Source: CAD feature listing. Evaluate the final solid. Frame: model axes, mm. Face numbers are marked on the shaded views. A direction names the side the tool comes from. Round coordinates to 2 decimals unless told otherwise and drop trailing zeros. Loops run counter-clockwise (first coordinate to the right, second up) from the corner with the lowest first, then second, coordinate; pieces in that order, holes last.
(1) Material intervals for probe 1 along X at (y, z) = (300, 0.75); probe 2 along Y at (x, z) = (4, 0.45); probe 3 along X at (y, z) = (301, 2.05), sorted ascending.
(2) Section A-A, the plane x = 4. Return the cut outline in (y, z), plus the area to 3 significant figures.
(3) Section B-B, the plane z = 2.75. Return the cut outline in (x, y) (3 decimals).
(4) First-contact query: pin 1 Ø4.5 at (x, y) = (2.5, 300) entering from +Z; pin 2 Ø1.7 at (x, y) = (-3, 300) entering from +Z. Flat tips, straight axial feed; report the tip coordinate or a pass-through.
(5) Section D-D, the plane x = 6.25. Return the cut outline in (y, z).
(6) Set-up query: the marked faces 1 and 2. Return all of +Z, -Z, +X, -X, +Y, -Y with unobstructed straight access to the full face (end or side cutting, diameter ignored); none if empty.
(7) Section C-C, the plane y = 298.75. Return the cut outline in (x, z), plus the area to 3 significant figures.
(8) Mould query, pull axis X, two halves, no side actions, for the marked faces 3, 4 and 5. Classes: pulls with the +X half, pulls with the -X half, needs draft (parallel to the pull), parting line crosses it, or undercut.
```python
from build123d import *

# Parameters (mm, degrees)
SKETCH_1_W                  = 18
SKETCH_1_H                  = 8
EXTRUDE_1_DEPTH             = 3
CUT_EXTRUDE_1_DEPTH         = 2
CUT_EXTRUDE_2_DEPTH         = 2
HOLE_WIZARD_3_6_3_6_1_D     = 3.6
HOLE_WIZARD_3_6_3_6_1_DEPTH = 3


with BuildPart() as part:
    # 草图1 → 凸台-拉伸1 (new body)
    with BuildSketch(Plane(origin=(0, 0, 0), x_dir=(-1, 0, 0), z_dir=(0, 0, -1))):
        with Locations((0, 300)):
            Rectangle(SKETCH_1_W, SKETCH_1_H)
    extrude(amount=-EXTRUDE_1_DEPTH)

    # 草图2 → 切除-拉伸1 (cut)
    with BuildSketch(Plane.XY.offset(3)):
        Polygon((-0.65, 300), (-2.325, 302.901185103), (-5.675, 302.901185103), (-7.35, 300), (-5.675, 297.098814897), (-2.325, 297.098814897), align=None)
    extrude(amount=-CUT_EXTRUDE_1_DEPTH, mode=Mode.SUBTRACT)

    # 草图3 → 切除-拉伸2 (cut)
    with BuildSketch(Plane.XY.offset(3)):
        Polygon((5.675, 297.098814897), (7.35, 300), (5.675, 302.901185103), (2.325, 302.901185103), (0.65, 300), (2.325, 297.098814897), align=None)
    extrude(amount=-CUT_EXTRUDE_2_DEPTH, mode=Mode.SUBTRACT)

    # Ø3.6 (3.6) 直径孔1
    with Locations(Plane(origin=(0, 0, 0), x_dir=(-1, 0, 0), z_dir=(0, 0, -1))):
        with Locations((-4, 300), (4, 300)):
            Hole(HOLE_WIZARD_3_6_3_6_1_D / 2, depth=HOLE_WIZARD_3_6_3_6_1_DEPTH)


solid = part.part
```
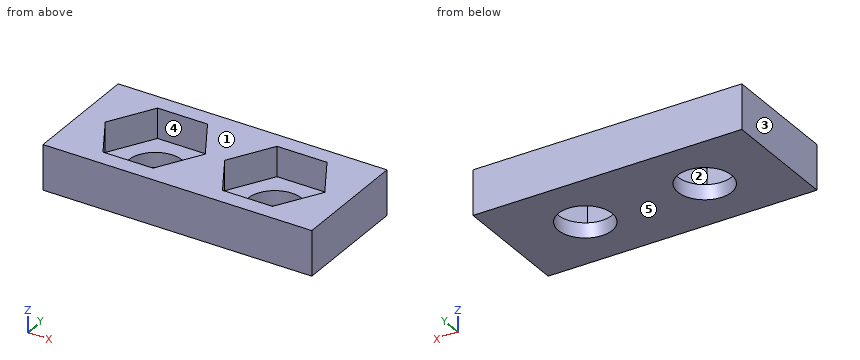
Output values:
1. probe 1: x = -9 to -5.8, -2.2 to 2.2, 5.8 to 9
1. probe 2: y = 296 to 298.2, 301.8 to 304
1. probe 3: x = -9 to -6.77, -1.23 to 1.23, 6.77 to 9
2. outline: (296, 0) - (298.2, 0) - (298.2, 1) - (297.1, 1) - (297.1, 3) - (296, 3) - close; (301.8, 0) - (304, 0) - (304, 3) - (302.9, 3) - (302.9, 1) - (301.8, 1) - close
2. area: 8.80 mm2
3. outline: (-9, 296) - (9, 296) - (9, 304) - (-9, 304) - close; hole (-7.35, 300) - (-5.675, 297.099) - (-2.325, 297.099) - (-0.65, 300) - (-2.325, 302.901) - (-5.675, 302.901) - close; hole (0.65, 300) - (2.325, 297.099) - (5.675, 297.099) - (7.35, 300) - (5.675, 302.901) - (2.325, 302.901) - close
4. pin 1: stops at z = 3
4. pin 2: stops at z = 1
5. outline: (296, 0) - (304, 0) - (304, 3) - (301.91, 3) - (301.91, 1) - (298.09, 1) - (298.09, 3) - (296, 3) - close
6. face 1: +Z, +X, -X, +Y, -Y
6. face 2: +Z
7. outline: (-9, 0) - (-5.3, 0) - (-5.3, 1) - (-6.63, 1) - (-6.63, 3) - (-9, 3) - close; (-2.7, 0) - (2.7, 0) - (2.7, 1) - (1.37, 1) - (1.37, 3) - (-1.37, 3) - (-1.37, 1) - (-2.7, 1) - close; (5.3, 0) - (9, 0) - (9, 3) - (6.63, 3) - (6.63, 1) - (5.3, 1) - close
7. area: 27.8 mm2
8. face 3: pulls with the -X half
8. face 4: undercut
8. face 5: needs draft
